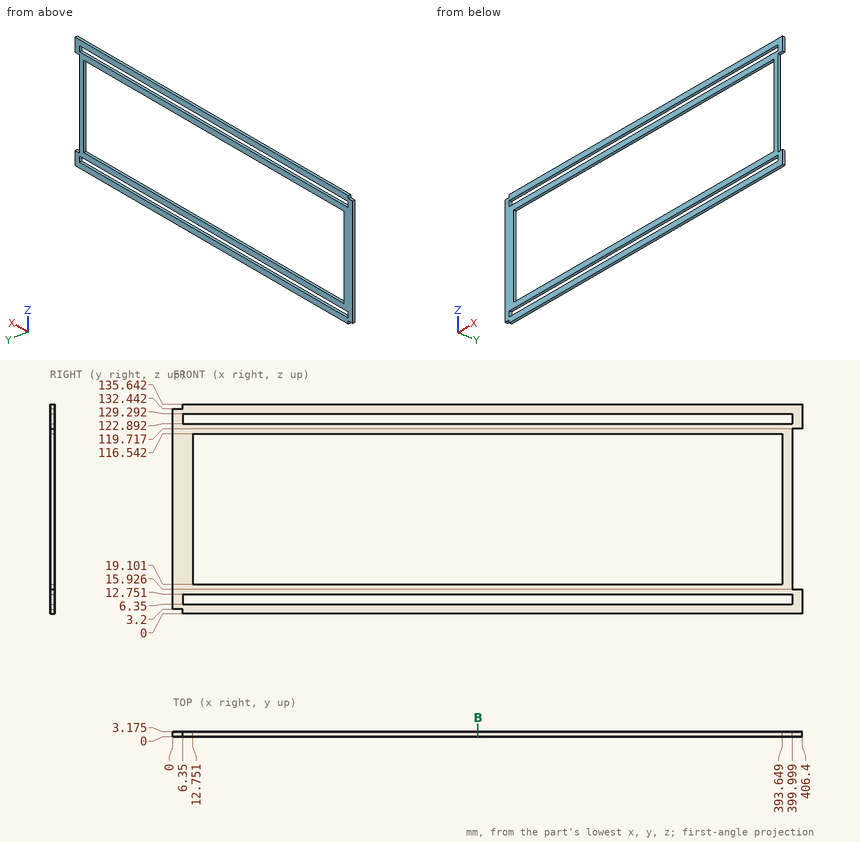
Part print with two shaded views. Sizes in mm from the minimum x, y, z corner. Round coordinates to 2 decimals unless told otherwise and drop trailing zeros. Use one line per item in the form item = value.
Item 1: Drill centre lines: line 1 (Z direction, x = 137, y = 0.2); line 2 (X direction, y = 0.2, z = 108.5); line 3 (X direction, y = 3.05, z = 8). Where is each one in solid material? Low to high.
Returned:
line_1 = 0 to 6.35, 12.75 to 19.1, 116.54 to 122.89, 129.29 to 135.64
line_2 = 0 to 12.75, 393.65 to 400
line_3 = 0 to 6.35, 400 to 406.4
Item 2: Cut at B-B, the plane x = 197. Give the number of separate pieces and of enclosed holes in the cut face.
Returned:
separate_pieces = 4
enclosed_holes = 0
Item 3: Flat gauge pins, fed straight in: pin 1 Ø1 at (y, z) = (1, 135) entering from -X; pin 2 Ø1 at (y, z) = (2.5, 92.5) entering from +X. Where does each tip first touch, or does it go through?
Returned:
pin_1 = 6.35
pin_2 = 400
